Input: part model. Units: mm. Frame: model coordinates. Face numbers are marked on the shaded views. A direction names the side the tool comes from. Round coordinates to 2 decimals unless told otherwise and drop trailing zeros. Order: outer loops, then holes, each group sorted by start corner. A loop starts at its lowest first (then second) coordinate and runs counter-clockwise, first axis right, second up. Notation, with made-up numbers: (61.5, 56) - (90.5, 56) arc R26 cw to (90.5, 79) - close; hole circle Ø1 at (35, -35.75). An arc over 180 degrees is marked (long way). One line per item, written item: value. Start each with the question number.
Autodesk Inventor part; units mm, degrees
ref_plane "YZ Plane" through (0, 0, 0) normal (1, 0, 0) x (0, 1, 0)
ref_plane "XZ Plane" through (0, 0, 0) normal (0, 1, 0) x (-1, 0, 0)
ref_plane "XY Plane" through (0, 0, 0) normal (0, 0, 1) x (1, 0, 0)
sketch "Sketch1" plane through (0, 0, 0) normal (0, 0, 1) x (1, 0, 0)
  circle A0 centre (0, 0) radius 4.15
  circle A1 centre (0, 0) radius 10
  dimension "d0" = 8.3
  dimension "d1" = 20
extrude "Extrusion1" add sketch "Sketch1" along normal blind 10
sketch "Sketch2" plane through (0, 0, 0) normal (1, 0, 0) x (0, 1, 0)
  line L0 (10, 0) -> (10, 10)
  line L1 (10, 0) -> (-10, 0)
  point P0 (0, 0)
  point P1 (0, 4)
  dimension "d22" = 4
hole "Hole1" at (0, 0, 4) direction (-1, 0, 0) diameter 2 end through all both
sketch "Sketch3" plane through (0, 0, 0) normal (0, 1, 0) x (-1, 0, 0)
  line L0 (10, 0) -> (-10, 0)
  point P0 (0, 0)
  point P1 (0, 4)
  dimension "d11" = 4
hole "Hole2" at (0, 0, 4) direction (0, 1, 0) diameter 2 end through all both
sketch "Sketch4" plane through (0, 0, 10) normal (0, 0, 1) x (1, 0, 0)
  circle A0 centre (0, 0) radius 10
  circle A1 centre (0, 0) radius 4.15
  circle A2 centre (0, 0) radius 6
  dimension "d21" = 12
extrude "Extrusion2" cut sketch "Sketch4" against normal blind 2 contours A0
properties part number "0008-30-008"
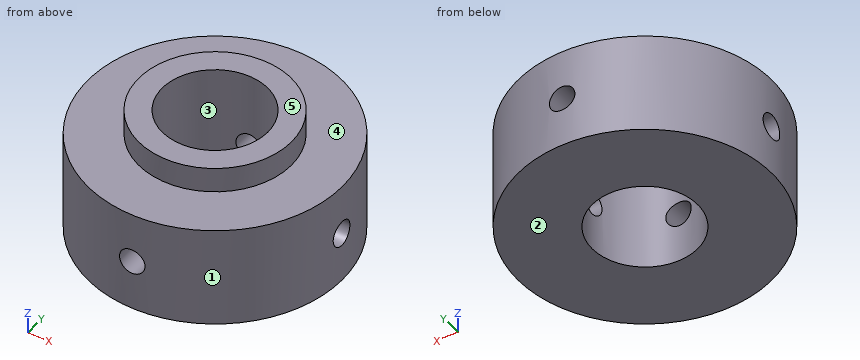
1. Set-up query: the marked faces 4 and 5. Return all of +Z, -Z, +X, -X, +Y, -Y with unobstructed straight access to the full face (end or side cutting, diameter ignored); none if empty.
2. Line query: line 1 (Y direction, x = 0, z = 7.75); line 2 (Z direction, x = 0, y = -7.45). Output: solid intervals per line, ascending. Write a range as from..to.
3. Pull-direction query (Y, two-part tool) for the marked faces 1, 2 and 3; classes: released by +Y, released by -Y, zero draft, split by the parting line, or undercut.
4. Section C-C (x = 8). Return the cut outline in (y, z), then the cut area to 3 significant figures.
5. Pin query (flat end, axial travel): pin 1 (1.6 mm diameter, centred on y = 0, z = 4, fed in from +X); pin 2 (4 mm diameter, centred on y = -3.5, z = 6, fed in from +X); pin 3 (4 mm diameter, centred on x = 5.5, z = 2, fed in from +Y); pin 4 (1.5 mm diameter, centred on y = 5, z = 4, fed in from -X). Return the tip coordinate at first contact, or that it passes through.
6. Section A-A (x = 0). Return the cut outline in (y, z).
7. Section D-D (z = 9.5). Return the cut outline in (x, y), then the cut area to 3 significant figures.
Solved:
1. face 4: +Z
1. face 5: +Z, +X, -X, +Y, -Y
2. line 1: y = -10..-4.15, 4.15..10
2. line 2: z = 0..3, 5..8
3. face 1: split by the parting line
3. face 2: zero draft
3. face 3: undercut
4. outline: (-6, 0) - (6, 0) - (6, 8) - (-6, 8) - close; hole circle Ø2 at (0, 4)
4. area: 92.9 mm²
5. pin 1: passes through
5. pin 2: stops at x = 9.89
5. pin 3: stops at y = 9.37
5. pin 4: stops at x = -9.05
6. outline: (-10, 0) - (-4.15, 0) - (-4.15, 3) - (-10, 3) - close; (-10, 5) - (-4.15, 5) - (-4.15, 10) - (-6, 10) - (-6, 8) - (-10, 8) - close; (4.15, 0) - (10, 0) - (10, 3) - (4.15, 3) - close; (4.15, 5) - (10, 5) - (10, 8) - (6, 8) - (6, 10) - (4.15, 10) - close
7. outline: circle Ø12 at (0, 0); hole circle Ø8.3 at (0, 0)
7. area: 59.0 mm²
